from build123d import *

# Parameters (mm, degrees)
BOSS_EXTRUDE1_DEPTH = 2
SKETCH2_R           = 3
SKETCH2_R_2         = 1.95
BOSS_EXTRUDE2_DEPTH = 12


with BuildPart() as part:
    # Sketch1 → Boss-Extrude1 (new body)
    with BuildSketch(Plane.XY):
        with BuildLine():
            Line((-33, -15), (33, -15))
            ThreePointArc((33, -15), (34.414213562, -14.414213562), (35, -13))
            Line((35, -13), (35, 13))
            ThreePointArc((35, 13), (34.414213562, 14.414213562), (33, 15))
            Line((33, 15), (-33, 15))
            ThreePointArc((-33, 15), (-34.414213562, 14.414213562), (-35, 13))
            Line((-35, 13), (-35, -13))
            ThreePointArc((-35, -13), (-34.414213562, -14.414213562), (-33, -15))
        make_face()
    extrude(amount=BOSS_EXTRUDE1_DEPTH)

    # Sketch2 → Boss-Extrude2 (add)
    # profile 1 of 4: a face of its own
    with BuildSketch(Plane(origin=(0, 0, 0), x_dir=(-1, 0, 0), z_dir=(0, 0, -1))):
        with Locations((28, -7.5)):
            Circle(SKETCH2_R)
        with Locations((28, -7.5)):
            Circle(SKETCH2_R_2, mode=Mode.SUBTRACT)
    # profile 2 of 4: a face of its own
    with BuildSketch(Plane(origin=(0, 0, 0), x_dir=(-1, 0, 0), z_dir=(0, 0, -1))):
        with Locations((30, 7.5)):
            Circle(SKETCH2_R)
        with Locations((30, 7.5)):
            Circle(SKETCH2_R_2, mode=Mode.SUBTRACT)
    # profile 3 of 4: a face of its own
    with BuildSketch(Plane(origin=(0, 0, 0), x_dir=(-1, 0, 0), z_dir=(0, 0, -1))):
        with Locations((-30, 7.5)):
            Circle(SKETCH2_R)
        with Locations((-30, 7.5)):
            Circle(SKETCH2_R_2, mode=Mode.SUBTRACT)
    # profile 4 of 4: a face of its own
    with BuildSketch(Plane(origin=(0, 0, 0), x_dir=(-1, 0, 0), z_dir=(0, 0, -1))):
        with Locations((-28, -7.5)):
            Circle(SKETCH2_R)
        with Locations((-28, -7.5)):
            Circle(SKETCH2_R_2, mode=Mode.SUBTRACT)
    extrude(amount=BOSS_EXTRUDE2_DEPTH)


solid = part.part
Work out the finished part from the listing and answer in its coordinate system (mm). A direction names the side the tool comes from. Round coordinates to 2 decimals unless told otherwise and drop trailing zeros. Write each loop counter-clockwise with the first axis right and the second up, starting at its lowest first coordinate (ties: lowest second). Pieces come first, ordered by that corner, then holes. Notation, with made-up numbers: (-36, 64) -> (16, 64) arc R11 ccw to (16, 82) -> close; hole circle Ø8 at (-0.5, -9). An arc over 180 degrees is marked (long way). Write each question's results on one line, items separated by ' | '.
Item 1: Flat-ended cylindrical pins translate along their axes: P1, Ø1, axis at x = -6.5, z = -1.5, coming from the -Y side; P2, Ø15, axis at x = -11.5, y = 2, coming from the -Z side; P3, Ø2, axis at x = -25.5, z = -3, coming from the +Y side; P4, Ø4, axis at y = -5.5, z = -2.5, coming from the -X side. Find the tip coordinate at first contact, or state that the pin passes through.
Result set:
P1: through | P2: z = 0 | P3: y = -4.9 | P4: x = -31
Item 2: Which of the six approach directions +Z, -Z, +X, -X, +Y, -Y give full straight-line access (tool end or side, diameter ignored) to faces 1 (the face through (34.43, 14.4, 0.99)), 2 (the face through (-28, -7, 0))?
Result set:
face 1: +Z, -Z, +X, +Y | face 2: -Z
Item 3: A cutting plane is placed at C-C, the plane x = 9. Determine the outline of the cut face in (y, z).
Result set:
outline: (-15, 0) -> (15, 0) -> (15, 2) -> (-15, 2) -> close
Item 4: A cutting plane is placed at A-A, the plane z = -9. Determine the outline of the cut face in (x, y).
Result set:
outline: circle Ø6 at (-30, 7.5); circle Ø6 at (-28, -7.5); circle Ø6 at (28, -7.5); circle Ø6 at (30, 7.5); hole circle Ø3.9 at (-30, 7.5); hole circle Ø3.9 at (-28, -7.5); hole circle Ø3.9 at (28, -7.5); hole circle Ø3.9 at (30, 7.5)
Item 5: A cutting plane is placed at B-B, the plane y = 7.5. Determine the outline of the cut face in (x, z).
Result set:
outline: (-35, 0) -> (-33, 0) -> (-33, -12) -> (-31.95, -12) -> (-31.95, 0) -> (-28.05, 0) -> (-28.05, -12) -> (-27, -12) -> (-27, 0) -> (27, 0) -> (27, -12) -> (28.05, -12) -> (28.05, 0) -> (31.95, 0) -> (31.95, -12) -> (33, -12) -> (33, 0) -> (35, 0) -> (35, 2) -> (-35, 2) -> close
Item 6: Find the intervals of material crossed by line 1 along Y through (x, z) = (30, -4.25); line 2 along Y through (x, z) = (28, -3.5); line 3 along X through (y, z) = (9.25, -6), in increasing order. Write a range as [from, to].
Result set:
line 1: [-9.74, -5.26], [4.5, 5.55], [9.45, 10.5] | line 2: [-10.5, -9.45], [-5.55, -4.5], [5.26, 9.74] | line 3: [-32.44, -30.86], [-29.14, -27.56], [27.56, 29.14], [30.86, 32.44]
